Work out the finished part from the listing and answer in its coordinate system (mm). A direction names the side the tool comes from. Give positions to 0.01 mm unless a question says otherwise; leave off trailing zeros. Loops run counter-clockwise (first coordinate to the right, second up) from the corner with the lowest first, then second, coordinate; pieces in that order, holes last. Notation, with made-up numbers: (88.25, -38) - (138.25, -38) arc R28 cw to (138.25, -15) - close; hole circle Ø11 at (30, 77.25). An arc over 180 degrees is marked (long way). Use CSV: the item, a comma, the result in double quotes.
from build123d import *

# Parameters (mm, degrees)
BOSS_EXTRUDE2_DEPTH = 4.7625


with BuildPart() as part:
    # Sketch1 → Boss-Extrude2 (new body)
    with BuildSketch(Plane(origin=(0, 0, 0), x_dir=(1, 0, 0), z_dir=(0, 1, 0))):
        Polygon((185.950525, 135.919), (185.950525, 147.9675), (6.09505, 147.968), (5.62377, 147.949), (5.15525, 147.894), (4.6936, 147.803), (4.24021, 147.675), (3.79786, 147.511), (3.37068, 147.314), (2.96003, 147.085), (2.56728, 146.822), (2.19797, 146.529), (1.85208, 146.21), (1.53238, 145.865), (1.24024, 145.495), (0.978408, 145.102), (0.748273, 144.691), (0.551215, 144.264), (0.38723, 143.822), (0.259071, 143.368), (0.168121, 142.907), (0.112999, 142.44), (0.0950846, 141.967), (0.0937066, 6.0923), (0.112999, 5.62102), (0.168121, 5.15387), (0.259071, 4.69085), (0.38723, 4.23746), (0.551215, 3.79511), (0.748273, 3.36793), (0.978408, 2.95727), (1.24024, 2.56453), (1.53238, 2.19659), (1.85208, 1.84933), (2.19797, 1.52962), (2.56728, 1.23748), (2.96003, 0.975653), (3.37068, 0.745518), (3.79786, 0.549836), (4.24021, 0.385851), (4.6936, 0.257693), (5.15525, 0.165365), (5.62377, 0.110243), (6.09505, 0.0909507), (185.950525, 0.0909507), (185.950525, 12.1405), (12.1447, 12.1405), (12.1447, 135.919), align=None)
        Polygon((5.10565, 7.5117), (5.58518, 7.75698), (6.11851, 7.84105), (6.65318, 7.75698), (7.13274, 7.5117), (7.51445, 7.12996), (7.75974, 6.65043), (7.8438, 6.11572), (7.75974, 5.5838), (7.51445, 5.10286), (7.13274, 4.72115), (6.65318, 4.47587), (6.11851, 4.3918), (5.58518, 4.47587), (5.10565, 4.72115), (4.72391, 5.10286), (4.47862, 5.5838), (4.39318, 6.11572), (4.47862, 6.65043), (4.72391, 7.12996), align=None, mode=Mode.SUBTRACT)
        Polygon((124.992, 7.5117), (125.473, 7.75698), (126.007, 7.84105), (126.54, 7.75698), (127.021, 7.5117), (127.403, 7.12996), (127.648, 6.65043), (127.732, 6.11572), (127.648, 5.5838), (127.403, 5.10286), (127.021, 4.72115), (126.54, 4.47587), (126.007, 4.3918), (125.473, 4.47587), (124.992, 4.72115), (124.612, 5.10286), (124.365, 5.5838), (124.281, 6.11572), (124.365, 6.65043), (124.612, 7.12996), align=None, mode=Mode.SUBTRACT)
        Polygon((5.10565, 143.338), (5.58518, 143.583), (6.11851, 143.667), (6.65318, 143.583), (7.13274, 143.338), (7.51445, 142.956), (7.75974, 142.477), (7.8438, 141.942), (7.75974, 141.409), (7.51445, 140.929), (7.13274, 140.547), (6.65318, 140.302), (6.11851, 140.217), (5.58518, 140.302), (5.10565, 140.547), (4.72391, 140.929), (4.47862, 141.409), (4.39318, 141.942), (4.47862, 142.477), (4.72391, 142.956), align=None, mode=Mode.SUBTRACT)
        Polygon((124.992, 143.338), (125.473, 143.583), (126.007, 143.667), (126.54, 143.583), (127.021, 143.338), (127.403, 142.956), (127.648, 142.477), (127.732, 141.942), (127.648, 141.409), (127.403, 140.929), (127.021, 140.547), (126.54, 140.302), (126.007, 140.217), (125.473, 140.302), (124.992, 140.547), (124.612, 140.929), (124.365, 141.409), (124.281, 141.942), (124.365, 142.477), (124.612, 142.956), align=None, mode=Mode.SUBTRACT)
    extrude(amount=BOSS_EXTRUDE2_DEPTH)


solid = part.part
Item 1: A cutting plane is placed at B-B on y = 4. State how many separate pieces and enclosed holes the cut face has, and give its area (3 significant figures).
Determined:
separate pieces,"1"
enclosed holes,"4"
area,"5,920 mm²"
Item 2: For faces 4 (the flat face through (100, 2, -12.14)), 5 (the flat face through (10, 4.762, -69)), determine the directions among +Z, -Z, +X, -X, +Y, -Y from which every point of the face is accessible in a straight line to the end or side of a thin tool.
Determined:
face 4,"+X, +Y, -Y"
face 5,"+Z, -Z, +X, -X, +Y"
Item 3: Find the intervals of material crossed by line 1 (Z direction, x = 21, y = 3.85); line 2 (X direction, y = 3.75, z = -7); line 3 (X direction, y = 2, z = -65.5), in increasing order.
Determined:
line 1,"z = -147.97 to -135.92, -12.14 to -0.09"
line 2,"x = 0.09 to 4.66, 7.58 to 124.55, 127.47 to 185.95"
line 3,"x = 0.09 to 12.14"
Item 4: Given P1, Ø1.4, axis at y = 2, z = -73.5, coming from the +X side, flat-ended and moving along its own axis, determine where the tip first touches the part or whether it passes through.
Determined:
P1,"stops at x = 12.14"
Item 5: A cutting plane is placed at D-D on z = -80. Determine the outline of the cut face in (x, y).
Determined:
outline,"(0.09, 0) - (12.14, 0) - (12.14, 4.76) - (0.09, 4.76) - close"
Item 6: A cutting plane is placed at A-A on x = 52. Determine the outline of the cut face in (y, z), and give its area (3 significant figures).
Determined:
outline,"(0, -147.97) - (4.76, -147.97) - (4.76, -135.92) - (0, -135.92) - close; (0, -12.14) - (4.76, -12.14) - (4.76, -0.09) - (0, -0.09) - close"
area,"115 mm²"
Item 7: The mould has two halves that part along Z. Classify faces 1 (the flat face through (12.145, 2, -73)), 2 (the flat face through (185.951, 2, -6)), 3 (the flat face through (95, 2, -0.091)): pulls with the +Z half, pulls with the -Z half, needs draft (parallel to the pull), parting line crosses it, or undercut.
Determined:
face 1,"undercut"
face 2,"needs draft"
face 3,"pulls with the +Z half"
